Read the model definition and answer for the solid it produces. Units are mm, in the model's axes. Face numbers are marked on the shaded views. A direction names the side the tool comes from. Round coordinates to 2 decimals unless told otherwise and drop trailing zeros. Write each loop counter-clockwise with the first axis right and the second up, starting at its lowest first coordinate (ties: lowest second). Pieces come first, ordered by that corner, then holes. Notation, with made-up numbers: (12, 34.5) - (68, 34.5) arc R36 ccw to (68, 69.5) - close; hole circle Ø11 at (-9, 5.25). An arc over 180 degrees is marked (long way). Use one line per item in the form item = value. Start each with the question number.
1) For the marked faces 1, 2 and 3, determine the directions among +Z, -Z, +X, -X, +Y, -Y from which every point of the face is accessible in a straight line to the end or side of a thin tool.
2) The part is cut by section C-C, the plane y = 40.5. Give the vertices of the cut face in (x, z), plus the area to 3 significant figures.
3) For a pull along Y with two mould halves and no side action, classify the marked faces 4, 5, 6 and 7 as released by +Y, released by -Y, zero draft, split by the parting line, or undercut.
4) Consider line 1 along Y through (x, z) = (-77, 21); line 2 along X through (y, z) = (22, 15.5); line 3 along X through (y, z) = (33, 10). Determine where each line is inside the solid, lowest interval first. Write a range as from..to.
5) The part is cut by section A-A, the plane y = -56.5. Give the vertices of the cut face in (x, z), plus the area to 3 significant figures.
6) The part is cut by section B-B, the plane z = 14.5. Give the vertices of the cut face in (x, y).
7) Each of these flat-tipped pins is pushed along its axis until it touches: pin 1 (3 mm diameter, centred on y = 45.5, z = 25.5, fed in from -X); pin 2 (8 mm diameter, centred on y = -28, z = 9, fed in from -X); pin 3 (1.5 mm diameter, centred on y = 0, z = 25, fed in from -X). Where does it stop, or does it pass through?
8) The part is cut by section D-D, the plane x = -68. Give the vertices of the cut face in (y, z).
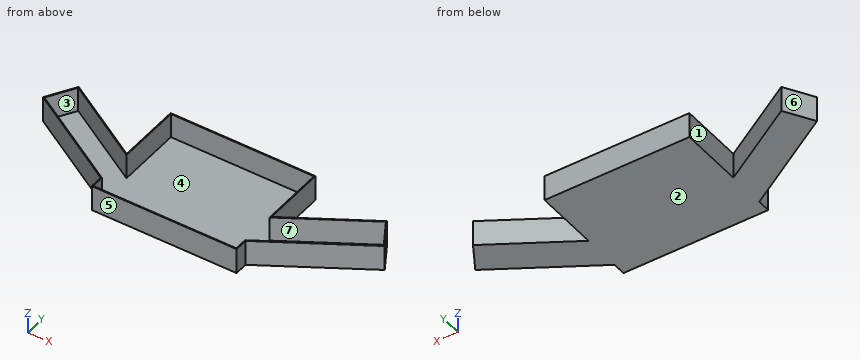
from build123d import *

# Parameters (mm, degrees)
F1_DEPTH = 30
F2_T     = -1


with BuildPart() as f1:
    # F0 (on Top) → F1 (new body)
    with BuildSketch(Plane.XY):
        Polygon((62.6864729471, -8.4317315359), (62.6864729471, 66.8668336705), (-107.3135270529, 66.8668336705), (-107.3135270529, 45.8668336705), (-107.3135270529, -8.4317315359), (-107.3135270529, -52.8148650094), (-107.3135270529, -68.1331663295), (62.6864729471, -68.1331663295), (62.6864729471, -52.8148650094), align=None)
        Polygon((158.6372393407, 49.4712554003), (62.6864729471, -8.4317315359), (62.6864729471, -52.8148650094), (178.2709213291, 16.9363736336), align=None)
        Polygon((-107.3135270529, -52.8148650094), (-107.3135270529, -8.4317315359), (-203.2642934464, 49.4712554003), (-222.8979754349, 16.9363736336), align=None)
    extrude(amount=F1_DEPTH)

    # F2
    f2_openings = [f1.faces().sort_by_distance(p)[0] for p in [
        (-22.313527, -0.247476, 30),
    ]]
    offset(amount=F2_T, openings=f2_openings, kind=Kind.INTERSECTION)


solid = f1.part
Geometry results:
q1.face_1 = +Z, -Z, +Y
q1.face_2 = -Z, +X, -X, +Y, -Y
q1.face_3 = +Z
q2.outline = (-208.68, 0) - (-188.4, 0) - (-188.4, 30) - (-190.33, 30) - (-190.33, 1) - (-207.51, 1) - (-207.51, 30) - (-208.68, 30) - close; (-107.31, 0) - (62.69, 0) - (62.69, 30) - (61.69, 30) - (61.69, 1) - (-106.31, 1) - (-106.31, 30) - (-107.31, 30) - close; (143.77, 0) - (164.05, 0) - (164.05, 30) - (162.88, 30) - (162.88, 1) - (145.71, 1) - (145.71, 30) - (143.77, 30) - close
q2.area = 449 mm2
q3.face_4 = undercut
q3.face_5 = released by -Y
q3.face_6 = released by +Y
q3.face_7 = undercut
q4.line_1 = -68.13..-67.13, 65.87..66.87
q4.line_2 = -219.84..-218.67, -159.68..-157.74, -107.31..-106.31, 61.69..62.69, 113.11..115.05, 174.05..175.22
q4.line_3 = -213.2..-212.04, -177.91..-175.97, -107.31..-106.31, 61.69..62.69, 131.34..133.28, 167.41..168.58
q5.outline = (-107.31, 0) - (62.69, 0) - (62.69, 30) - (61.69, 30) - (61.69, 1) - (-106.31, 1) - (-106.31, 30) - (-107.31, 30) - close
q5.area = 228 mm2
q6.outline = (-222.9, 16.94) - (-107.31, -52.81) - (-107.31, -68.13) - (62.69, -68.13) - (62.69, -52.81) - (178.27, 16.94) - (158.64, 49.47) - (62.69, -8.43) - (62.69, 66.87) - (-107.31, 66.87) - (-107.31, -8.43) - (-203.26, 49.47) - close; hole (-221.53, 17.28) - (-106.31, -52.25) - (-106.31, -67.13) - (61.69, -67.13) - (61.69, -52.25) - (176.9, 17.28) - (158.3, 48.1) - (61.69, -10.2) - (61.69, 65.87) - (-106.31, 65.87) - (-106.31, -10.2) - (-202.92, 48.1) - close
q7.pin_1 = -206.57
q7.pin_2 = -155.06
q7.pin_3 = -196.08
q8.outline = (-68.13, 0) - (66.87, 0) - (66.87, 30) - (65.87, 30) - (65.87, 1) - (-67.13, 1) - (-67.13, 30) - (-68.13, 30) - close
